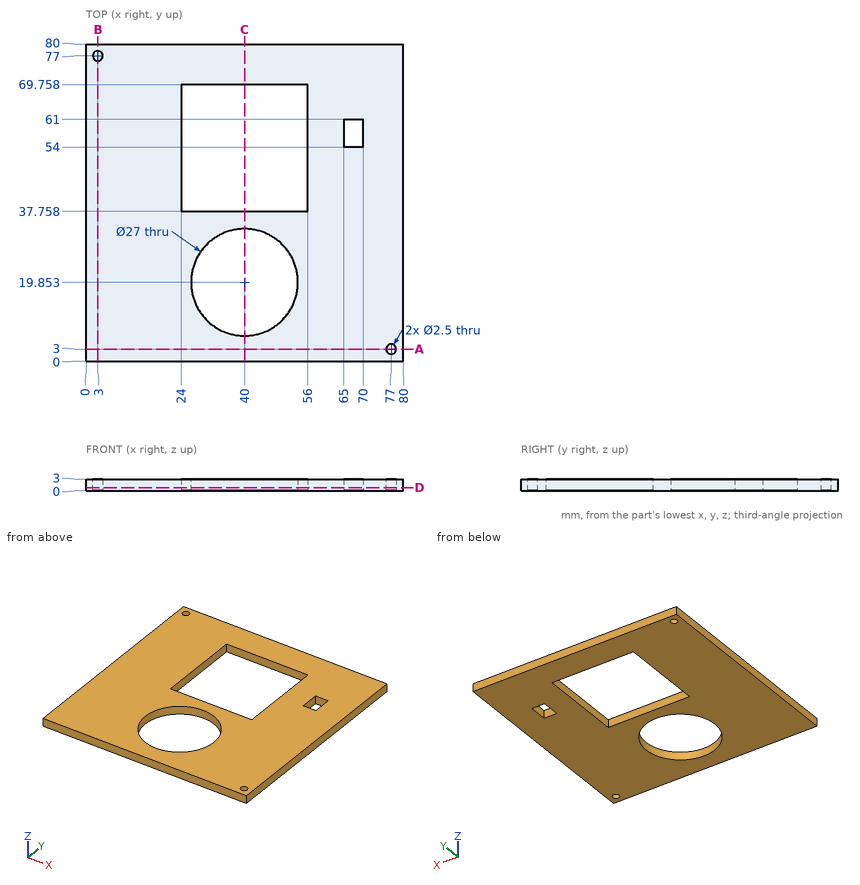
Design review of the part shown in the three views and the two pictorial views. Dimensions are in mm from the part's minimum x, y and z. Coordinates: 2 decimals unless noted, no trailing zeros. Loops run counter-clockwise (first coordinate to the right, second up) from the corner with the lowest first, then second, coordinate; pieces in that order, holes last. Notation, with made-up numbers: (15, -10) - (47, -10) arc R15 ccw to (47, 0) - close; hole circle Ø8 at (-29, -30.5). An arc over 180 degrees is marked (long way). Use a Markdown table: item, result. Add a question column.
Item 1: We need section C-C (x = 40). Give the boundary of the cut face in (y, z).
Item 2: Insertion check: pin 1 Ø8 at (x, y) = (51, 45.5) entering from +Z. The pin has a flat end and moves straight along its axis. Give the tip position at first contact, or say it passes through.
Item 3: For line 1 (Y direction, x = 40, z = 0.75); line 2 (X direction, y = 59, z = 1.2); line 3 (Y direction, x = 25, z = 2.35), list the stretches that pass through material, from the lowest coordinate up.
Item 4: We need section D-D (z = 0.85). Give the boundary of the cut face in (x, y).
Item 5: We need section A-A (y = 3). Give the boundary of the cut face in (x, z).
Results list:
| question | item | result |
|---|---|---|
| 1 | outline | (0, 0) - (6.35, 0) - (6.35, 3) - (0, 3) - close; (33.35, 0) - (37.76, 0) - (37.76, 3) - (33.35, 3) - close; (69.76, 0) - (80, 0) - (80, 3) - (69.76, 3) - close |
| 2 | pin 1 | passes through |
| 3 | line 1 | y = 0 to 6.35, 33.35 to 37.76, 69.76 to 80 |
| 3 | line 2 | x = 0 to 24, 56 to 65, 70 to 80 |
| 3 | line 3 | y = 0 to 37.76, 69.76 to 80 |
| 4 | outline | (0, 0) - (80, 0) - (80, 80) - (0, 80) - close; hole circle Ø2.5 at (3, 77); hole (24, 37.76) - (56, 37.76) - (56, 69.76) - (24, 69.76) - close; hole circle Ø27 at (40, 19.85); hole (65, 54) - (70, 54) - (70, 61) - (65, 61) - close; hole circle Ø2.5 at (77, 3) |
| 5 | outline | (0, 0) - (75.75, 0) - (75.75, 3) - (0, 3) - close; (78.25, 0) - (80, 0) - (80, 3) - (78.25, 3) - close |
